Verification items for this drawing (mm, ordinates from the low corner). A direction names the side the tool comes from. Give positions to 0.01 mm unless a question says otherwise; leave off trailing zeros. Write each loop counter-clockwise with the first axis right and the second up, starting at its lowest first coordinate (ties: lowest second). Pieces come first, ordered by that corner, then holes. Notation, with made-up numbers: M 53,31 L 98,31 A18 cw 98,37 Z; hole C 56,28.25 d10. An arc over 180 degrees is marked long. Write each question's results on one line, items separated by ' | '.
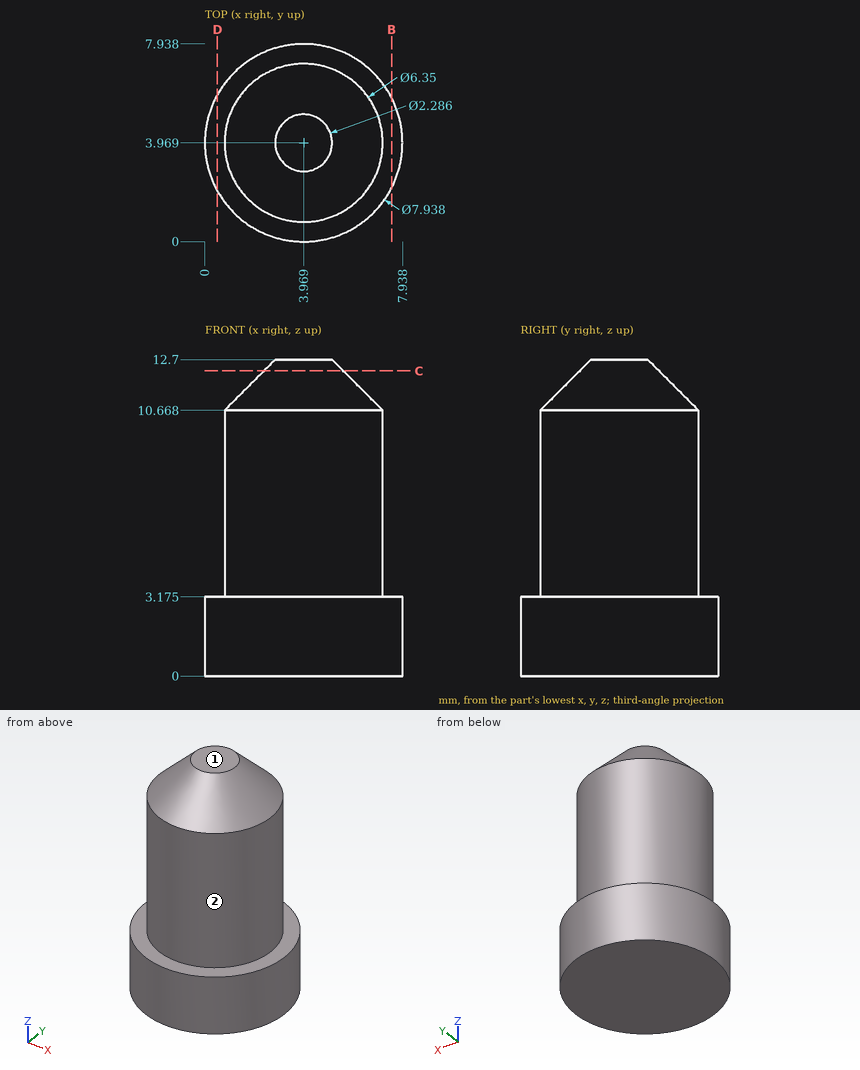
Q1. Section check D-D (x = 0.5). Enter the section's corners in (y, z) (1 decimal).
Answer key:
outline: M 2,0 L 5.9,0 L 5.9,3.2 L 2,3.2 Z
Q2. Material ranges on probe 1 along Z at (x, y) = (5.75, 6.75) (1 decimal); probe 2 along Y at (x, z) = (5.75, 9) (1 decimal); probe 3 along Y at (x, z) = (4, 5.5), recorded low to high. Write a range as [from, to].
Answer key:
probe 1: z = [0, 3.2] | probe 2: y = [1.3, 6.6] | probe 3: y = [0.79, 7.14]
Q3. Access from +Z, -Z, +X, -X, +Y, -Y to the whole of each face (thin tool, end or side, straight path). Record for the marked faces 1 and 2.
Answer key:
face 1: +Z, +X, -X, +Y, -Y | face 2: +Z
Q4. Section check C-C (z = 12.25). Enter the section's corners in (x, y) (1 decimal).
Answer key:
outline: C 4,4 d3.2
Q5. Section check B-B (x = 7.5). Enter the section's corners in (y, z) (1 decimal).
Answer key:
outline: M 2.2,0 L 5.8,0 L 5.8,3.2 L 2.2,3.2 Z
Q6. Depth check by flat-ended pin: P1, Ø3, axis at x = 2.5, z = 7.5, coming from the +Y side; P2, Ø1, axis at x = 2, z = 8, coming from the -Y side (1 decimal); P3, Ø1.5, axis at x = 4.5, z = 9.5, coming from the -Y side; P4, Ø2.5, axis at x = 5.5, y = 5.5, coming from the +Z side. Enter the tip coordinate at first touch or a pass-through.
Answer key:
P1: stops at y = 7.14 | P2: stops at y = 1.2 | P3: stops at y = 0.79 | P4: stops at z = 12.7
